from build123d import *

# Parameters (mm, degrees)
F1_DEPTH    = 355.6
F2_W        = 355.6
F2_H        = 76.2
F3_DEPTH    = 127
F5_DEPTH    = 457.201
F6_DEPTH    = 101.601
F7_T        = 3.175
F7_T3_DEPTH = 82.55
F7_T5_DEPTH = 361.95
F8_W        = 101.6
F8_H        = 228.6
F9_DEPTH    = 25.4


# Not quite as in the source:
# - a shell that OpenCascade refuses in one call is made with other operations: the cavity is built on its own and cut out


with BuildPart() as f1:
    # F0 (on Right) → F1 (new body)
    with BuildSketch(Plane.YZ):
        Polygon((0, 152.4), (0, 0), (76.2, 0), (76.2, 76.2), (76.2, 152.4), align=None)
        Polygon((76.2, 152.4), (76.2, 76.2), (127, 152.4), align=None)
    extrude(amount=F1_DEPTH)

    # F2 (on face) → F3 (join)
    with BuildSketch(Plane.XZ):
        Polygon((457.2, 152.4), (355.6, 152.4), (355.6, 76.2), align=None)
        Polygon((0, 76.2), (0, 152.4), (-101.6, 152.4), align=None)
        with Locations((177.8, 114.3)):
            Rectangle(F2_W, F2_H)
    extrude(amount=-F3_DEPTH)

    # F4 (on face) → F5 (cut, through all)
    with BuildSketch(Plane.YZ.offset(355.6)):
        Polygon((76.2, 76.2), (127, 76.2), (127, 152.4), align=None)
    extrude(amount=-F5_DEPTH, mode=Mode.SUBTRACT)

    # F4 (on face) → F6 (cut, through all)
    with BuildSketch(Plane.YZ.offset(355.6)):
        Polygon((76.2, 76.2), (127, 76.2), (127, 152.4), align=None)
    extrude(amount=F6_DEPTH, mode=Mode.SUBTRACT)

    # F7: shell of thickness 3.175, made by hand


with BuildPart() as f7_core1:
    # F7_t2: copy of F1
    add(f1.part)

    # the walls: a layer under each face that stays
    f7_faces = [f7_core1.faces().sort_by_distance(p)[0] for p in [
        (177.8, 0, 76.2),
        (-50.8, 63.5, 114.3),
        (177.8, 101.6, 114.3),
        (177.8, 76.2, 38.1),
        (0, 38.1, 38.1),
        (355.6, 38.1, 38.1),
        (406.4, 63.5, 114.3),
    ]]
    thicken(f7_faces, amount=-F7_T, mode=Mode.SUBTRACT)

    # F7_s4 → F7_t3 (cut)
    with BuildSketch(Plane.XZ.offset(-79.375)):
        Polygon((-0.0508, 76.1746), (1.905, 78.74), (3.175, 77.7875), (3.175, 76.2), align=None)
        Polygon((355.6508, 76.1746), (352.425, 76.2), (352.425, 77.7875), (353.695, 78.74), align=None)
    extrude(amount=F7_T3_DEPTH, mode=Mode.SUBTRACT)

    # F7_s6 → F7_t5 (cut)
    with BuildSketch(Plane.YZ.offset(-3.175)):
        Polygon((76.2581675968, 76.1823882688), (73.5582403155, 77.961173123), (73.025, 77.1613126498), (73.025, 76.2), align=None)
    extrude(amount=F7_T5_DEPTH, mode=Mode.SUBTRACT)


with BuildPart() as f1_1:
    add(f1.part)

    # what is left inside the walls is the cavity
    f7_cavity = [f7_core1.part.solids().sort_by_distance(p)[0] for p in [
        (269.169444, 63.179562, 152.36825),
    ]]
    add(f7_cavity, mode=Mode.SUBTRACT)

    # F8 (on face) → F9 (cut)
    with BuildSketch(Plane.XZ):
        with Locations((177.8, 38.1)):
            Rectangle(F8_W, F8_H)
    extrude(amount=-F9_DEPTH, mode=Mode.SUBTRACT)


solid = f1_1.part
Design review of the part built by this model. Coordinates are the model's own, in mm. A direction names the side the tool comes from. Round coordinates to 2 decimals unless told otherwise and drop trailing zeros. Order: outer loops, then holes, each group sorted by start corner. A loop starts at its lowest first (then second) coordinate and runs counter-clockwise, first axis right, second up.
1) Machinability: for faces 1 (the flat face through (-47.263, 49.005, 115.616)), 2 (the flat face through (352.425, 38, 39)), 3 (the flat face through (175, 76.2, 38)), which of the approach directions +Z, -Z, +X, -X, +Y, -Y give a long, thin tool a straight path to every point of the face, cutting with its end or side? Answer none if there is none.
The answers:
face 1: +Z
face 2: +Z, -Z
face 3: -Z, +X, -X, +Y
2) Draft analysis for pull direction X (two halves, no side actions). For faces 4 (the flat face through (0, 38, 39)), 5 (the flat face through (173.888, 101.956, 114.833)), 6 (the flat face through (314, 3.175, 94)), state which applies: released by +X, released by -X, zero draft, split by the parting line, or undercut.
The answers:
face 4: released by -X
face 5: zero draft
face 6: undercut
3) Consider section A-A (y = 30). State the section outline as (x, z) points (1 decimal), plus the area to 3 significant figures.
The answers:
outline: (-101.6, 152.4) - (0, 76.2) - (0, 0) - (3.2, 0) - (3.2, 77.8) - (-96.3, 152.4) - close; (352.4, 0) - (355.6, 0) - (355.6, 76.2) - (457.2, 152.4) - (451.9, 152.4) - (352.4, 77.8) - close
area: 1,290 mm2
4) Clearance check with flat-ended pins moving along their axes: pin 1 Ø6 at (x, y) = (391.5, 19.5) entering from +Z; pin 2 Ø8 at (y, z) = (86, 107.5) entering from +X; pin 3 Ø1 at (x, z) = (131.5, 86.5) entering from -Y. State where each tip first meets the part, or that it passes through.
The answers:
pin 1: stops at z = 109.34
pin 2: stops at x = 402.67
pin 3: stops at y = 78.92
5) Consider section C-C (x = 173.5). State the section outline as (y, z) points (3 decimals).
The answers:
outline: (73.025, 0) - (76.2, 0) - (76.2, 76.2) - (127, 152.4) - (123.184, 152.4) - (73.025, 77.161) - close
6) For L1, parallel to X at y = 41, z = 66 (3 decimals); L2, parallel to Y at x = 341, z = 40 (3 decimals); L3, parallel to X at y = 84, z = 116.5, list the stretches that pass through material, from the lowest coordinate up.
The answers:
L1: x = 0 to 3.175, 352.425 to 355.6
L2: y = 0 to 3.175, 73.025 to 76.2
L3: x = -53.73 to -48.44, 404.04 to 409.33
7) Consider section D-D (y = 95.5). State the section outline as (x, z) points.
The answers:
outline: (-101.6, 152.4) - (-38.6, 105.15) - (394.2, 105.15) - (457.2, 152.4) - (451.91, 152.4) - (396.54, 110.87) - (-40.94, 110.87) - (-96.31, 152.4) - close
8) Consider section B-B (x = 302). State the section outline as (y, z) points (3 decimals), plus the area to 3 significant figures.
The answers:
outline: (0, 0) - (3.175, 0) - (3.175, 152.4) - (0, 152.4) - close; (73.025, 0) - (76.2, 0) - (76.2, 76.2) - (127, 152.4) - (123.184, 152.4) - (73.025, 77.161) - close
area: 1,020 mm2
